The model under review builds one solid part; all positions refer to its coordinate system, in mm. Round coordinates to 2 decimals unless told otherwise and drop trailing zeros. Loops run counter-clockwise (first coordinate to the right, second up) from the corner with the lowest first, then second, coordinate; pieces in that order, holes last. Notation, with made-up numbers: M 14,-37 L 42,-37 A21 cw 42,-19 Z; hole C -19.75,39 d6. An arc over 180 degrees is marked long. Return JSON: item names as keys, results as strings. Group by question number.
Q1. To check wall thickness, follow line 1 along Z through (x, y) = (0, 1.7); line 2 along X through (y, z) = (4.75, 40). State the ranges of each line that lie inside material, in increasing order.
Q2. Consider section A-A (z = 0). State the section outline as (x, y) points, and give its area (3 significant figures).
Q3. Consider section B-B (x = 0). State the section outline as (y, z) points.
Autodesk Inventor part; units mm, degrees
ref_plane "YZ Plane" through (0, 0, 0) normal (1, 0, 0) x (0, 1, 0)
ref_plane "XZ Plane" through (0, 0, 0) normal (0, 1, 0) x (-1, 0, 0)
ref_plane "XY Plane" through (0, 0, 0) normal (0, 0, 1) x (1, 0, 0)
sketch "Sketch1" plane through (0, 0, 0) normal (0, 1, 0) x (-1, 0, 0)
  circle A0 centre (0, 0) radius 438.1 construction
  line L0 (500, -500) -> (-500, -500)
  line L1 (-500, -500) -> (-500, 500)
  line L2 (-500, 500) -> (500, 500)
  line L3 (500, 500) -> (500, -500)
  line L4 (0, -248.7708) -> (0, 248.7708) construction
  line L5 (-1768.3221, 0) -> (1768.3221, 0) construction
  circle A1 centre (0, 0) radius 50
  dimension "d0" = 876.2
  dimension "d1" = 1000
  dimension "d2" = 1000
  dimension "d5" = 100
extrude "Extrusion1" add sketch "Sketch1" along normal blind 5
properties part number "StatorGroundPlate"
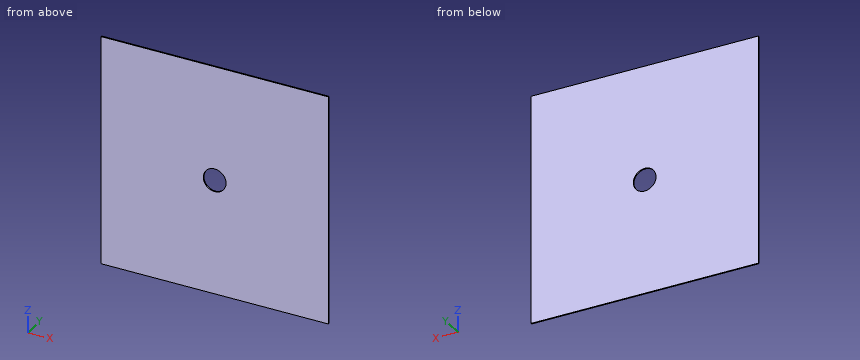
Values:
{
 "1": {"line 1": "z = -500 to -50, 50 to 500", "line 2": "x = -500 to -30, 30 to 500"},
 "2": {"outline": "M -500,0 L -50,0 L -50,5 L -500,5 Z; M 50,0 L 500,0 L 500,5 L 50,5 Z", "area": "4,500 mm2"},
 "3": {"outline": "M 0,-500 L 5,-500 L 5,-50 L 0,-50 Z; M 0,50 L 5,50 L 5,500 L 0,500 Z"}
}
